```python
from build123d import *

# Parameters (mm, degrees)
F0_R     = 4.25
F0_R_2   = 11.5
F0_R_3   = 6.5
F1_DEPTH = 5


with BuildPart() as f1:
    # F0 (on Top) → F1 (new body)
    with BuildSketch(Plane.XY):
        with BuildLine():
            Line((24.217633, -2.15), (24.217633, 14))
            Line((24.217633, 14), (-15.781855, 14))
            Line((-15.781855, 14), (-25.782367, 14))
            Line((-25.782367, 14), (-25.782367, -8.325128))
            ThreePointArc((-25.782367, -8.325128), (-12.029825, -17.702051), (4.285203, -21.000373))
            ThreePointArc((4.285203, -21.000373), (17.992916, -15.531456), (24.217633, -2.15))
        make_face()
        with Locations((-15.782367, -2.15)):
            Circle(F0_R, mode=Mode.SUBTRACT)
        with Locations((4.217633, -2.15)):
            Circle(F0_R_2, mode=Mode.SUBTRACT)
        with Locations((4.217633, -2.15)):
            Circle(F0_R_2)
        with Locations((4.217633, -2.15)):
            Circle(F0_R_3, mode=Mode.SUBTRACT)
    extrude(amount=-F1_DEPTH)


solid = f1.part
```
Part model, mm, in its own coordinate system. Coordinates: 2 decimals unless noted, no trailing zeros. Write each loop counter-clockwise with the first axis right and the second up, starting at its lowest first coordinate (ties: lowest second). Pieces come first, ordered by that corner, then holes.
Item 1: Slice it at D-D (x = 7). Write the cut outline in (y, z), and give its area (3 significant figures).
Item 2: Slice it at B-B (z = -2.2). Write the cut outline in (x, y), and give its area (3 significant figures).
Item 3: Slice it at C-C (x = -13.5). Write the cut outline in (y, z), and give its area (3 significant figures).
Item 4: Probe line 1 (X direction, y = -4.5, z = -3.2); line 2 (X direction, y = -2.5, z = -3.2); line 3 (X direction, y = -8, z = -4.7). List the from-to ranges inside material, lowest first.
Item 5: Slice it at A-A (y = -1.5). Write the cut outline in (x, z), and give its area (3 significant figures).
Item 6: Mould opens along Y. For faces 1 (the face through (-0.941, -6.105, -2.465)), 2 (the face through (-1, -7, 0)), 3 (the face through (0, 14, -2)) say: released by +Y, released by -Y, zero draft, split by the parting line, or undercut.
Results found:
1. outline: (-20.81, -5) - (-8.02, -5) - (-8.02, 0) - (-20.81, 0) - close; (3.72, -5) - (14, -5) - (14, 0) - (3.72, 0) - close
1. area: 115 mm2
2. outline: (-25.78, -8.33) arc R42 ccw to (4.29, -21) arc R20 ccw to (24.22, -2.15) - (24.22, 14) - (-25.78, 14) - close; hole circle Ø8.5 at (-15.78, -2.15); hole circle Ø13 at (4.22, -2.15)
2. area: 1,360 mm2
3. outline: (-17.05, -5) - (-5.74, -5) - (-5.74, 0) - (-17.05, 0) - close; (1.44, -5) - (14, -5) - (14, 0) - (1.44, 0) - close
3. area: 119 mm2
4. line 1: x = -25.78 to -19.32, -12.24 to -1.84, 10.28 to 23.94
4. line 2: x = -25.78 to -20.02, -11.55 to -2.27, 10.71 to 24.19
4. line 3: x = -25.78 to 1.38, 7.05 to 22.99
5. outline: (-25.78, -5) - (-19.98, -5) - (-19.98, 0) - (-25.78, 0) - close; (-11.58, -5) - (-2.25, -5) - (-2.25, 0) - (-11.58, 0) - close; (10.69, -5) - (24.22, -5) - (24.22, 0) - (10.69, 0) - close
5. area: 143 mm2
6. face 1: undercut
6. face 2: zero draft
6. face 3: released by +Y
